The model under review builds one solid part; all positions refer to its coordinate system, in mm. Face numbers are marked on the shaded views. A direction names the side the tool comes from. Round coordinates to 2 decimals unless told otherwise and drop trailing zeros. Order: outer loops, then holes, each group sorted by start corner. A loop starts at its lowest first (then second) coordinate and runs counter-clockwise, first axis right, second up. Notation, with made-up numbers: (48, -6.5) - (70, -6.5) arc R28 ccw to (70, 24.5) - close; hole circle Ø10 at (37.5, 50). An arc over 180 degrees is marked (long way). One line per question, with ' | ' between items. Start each with the question number.
Item 1: Add section C-C on z = 8. State the section outline as (x, y) points.
Item 2: Insertion check: pin 1 Ø6.5 at (x, y) = (-1, 23.5) entering from +Z; pin 2 Ø2 at (y, z) = (4, 7) entering from -X; pin 3 Ø1.5 at (y, z) = (6, 5) entering from -X. Each pin has a flat end and moves straight along its axis. Give the tip position at first contact, or say it passes through.
Item 3: Add section A-A on x = 0. State the section outline as (y, z) points, and give its area (3 significant figures).
Item 4: Draft analysis for pull direction Z (two halves, no side actions). For the marked faces 1, 2 and 3, state which applies: +Z half, -Z half, draft (parallel to the pull), parting line (faces both ways), or undercut.
Item 5: For L1, parallel to Z at x = 5.7, y = 3.85; L2, parallel to Y at x = 3.5, z = 9; L3, parallel to Y at x = 4.25, z = 4, list the stretches that pass through material, from the lowest coordinate up. Write a range as [from, to].
Item 6: Add section D-D on y = 30. State the section outline as (x, z) points.
Item 7: Tool access review of the marked faces 4 and 5: name each direction out of +Z, -Z, +X, -X, +Y, -Y from which nothing blocks a thin tool from reaching the whole face with its end or side.
Autodesk Inventor part; units mm, degrees
ref_plane "YZ Plane" through (0, 0, 0) normal (1, 0, 0) x (0, 1, 0)
ref_plane "XZ Plane" through (0, 0, 0) normal (0, 1, 0) x (-1, 0, 0)
ref_plane "XY Plane" through (0, 0, 0) normal (0, 0, 1) x (1, 0, 0)
sketch "Sketch1" plane through (0, 0, 0) normal (0, 0, 1) x (1, 0, 0)
  circle A0 centre (0, 25) radius 4.1
  circle A1 centre (0, 25) radius 15
  line L0 (-14.9332, 23.5861) -> (-12.7, 0)
  line L1 (-12.7, 0) -> (0, 0)
  line L2 (0, 0) -> (0, 25)
  line L3 (14.9332, 23.5861) -> (12.7, 0)
  line L4 (12.7, 0) -> (0, 0)
  circle A2 centre (0, 25) radius 11.15
  point P0 (14.9332, 23.5861)
  dimension "d1" = 30
  dimension "d0" = 8.2
  dimension "d2" = 25.4
  dimension "d5" = 25
  dimension "d16" = 22.3
extrude "Extrusion1" add sketch "Sketch1" along normal blind 10 contours A2 | A1 | A1 L3 L4 L2 | L2 L1 L0 A1
sketch "Sketch2" plane through (-12.7, 0, 0) normal (0, -1, 0) x (1, 0, 0)
  line L0 (0, 0) -> (25.4, 0)
  line L1 (25.4, 0) -> (25.4, 10)
  line L2 (0, 10) -> (25.4, 10)
  line L3 (0, 0) -> (0, 10)
  circle A0 centre (7, 5) radius 1.65
  point P0 (12.7, 0)
  point P1 (0, 5)
  dimension "d6" = 3.3
  dimension "d7" = 7
extrude "Extrusion2" cut sketch "Sketch2" against normal blind 15 contours A0
ref_plane "Work Plane1" through (-12.7, 5, 0) normal (0, -1, 0) x (1, 0, 0)
sketch "Sketch3" plane through (-12.7, 5, 0) normal (0, -1, 0) x (1, 0, 0)
  circle A0 centre (7, 5) radius 1.65
  line L0 (9.9, 6.6743) -> (9.9, 3.3257)
  line L1 (9.9, 3.3257) -> (7, 1.6514)
  line L2 (7, 1.6514) -> (4.1, 3.3257)
  line L3 (4.1, 3.3257) -> (4.1, 6.6743)
  line L4 (4.1, 6.6743) -> (7, 8.3486)
  line L5 (7, 8.3486) -> (9.9, 6.6743)
  line L6 (4.1, 6.6743) -> (9.9, 6.6743)
  line L7 (9.9, 6.6743) -> (9.9, 13.9222)
  line L8 (9.9, 13.9222) -> (4.1, 13.9222)
  line L9 (4.1, 13.9222) -> (4.1, 6.6743)
  point P0 (12.7, 0)
  dimension "d11" = 5.8
extrude "Extrusion3" cut sketch "Sketch3" against normal blind 3
mirror "Mirror1" about plane through (0, 0, 0) normal (1, 0, 0) of "Extrusion3", "Extrusion2"
sketch "Sketch4" plane through (0, 0, 0) normal (0, 0, -1) x (-1, 0, 0)
  line L0 (12.7, 0) -> (-12.7, 0)
  line L1 (14.9332, 23.5861) -> (12.7, 0)
  arc A0 (14.9332, 23.5861) -> (-14.9332, 23.5861) centre (0, 25) ccw
  line L2 (-12.7, 0) -> (-14.9332, 23.5861)
  circle A1 centre (0, 25) radius 4.1
  point P0 (0, 0)
extrude "Extrusion4" add sketch "Sketch4" against normal blind 3 contours A1
sketch "Sketch5" plane through (0, 0, 10) normal (0, 0, 1) x (1, 0, 0)
  line L0 (8.6, 8) -> (8.6, 5)
  line L1 (8.6, 5) -> (2.8, 5)
  line L2 (2.8, 5) -> (2.8, 8)
  line L3 (2.8, 8) -> (8.6, 8)
  line L4 (-8.6, 5) -> (-8.6, 8)
  line L5 (-8.6, 8) -> (-2.8, 8)
  line L6 (-2.8, 8) -> (-2.8, 5)
  line L7 (-2.8, 5) -> (-8.6, 5)
  line L8 (-12.7, 0) -> (12.7, 0)
  line L9 (12.7, 0) -> (14.9332, 23.5861)
  arc A0 (14.9332, 23.5861) -> (-14.9332, 23.5861) centre (0, 25) ccw
  line L10 (-14.9332, 23.5861) -> (-12.7, 0)
  circle A1 centre (0, 25) radius 4.1
  circle A2 centre (0, 25) radius 4.1
  circle A3 centre (0, 25) radius 11.15
  point P0 (0, 0)
  dimension "d17" = 22.3
extrude "Extrusion5" cut sketch "Sketch5" against normal blind 7 contours A3
properties part number "OTRO_EXTREMO" material "Steel, Mild, Welded"
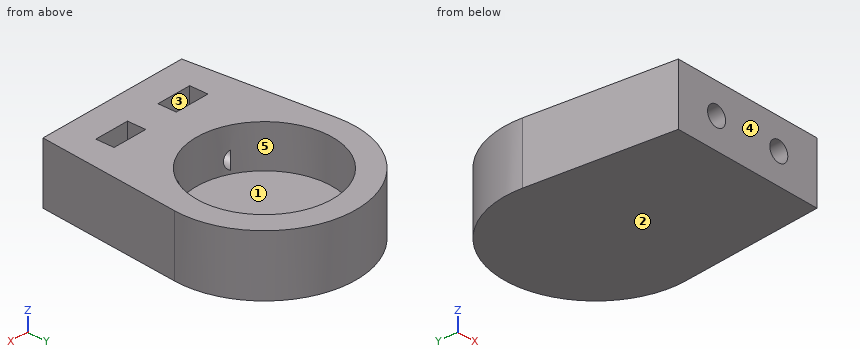
Determined:
1) outline: (-14.93, 23.59) - (-12.7, 0) - (12.7, 0) - (14.93, 23.59) arc R15 ccw (long way) to start; hole circle Ø22.3 at (0, 25); hole (-8.6, 5) - (-2.8, 5) - (-2.8, 8) - (-8.6, 8) - close; hole (2.8, 5) - (8.6, 5) - (8.6, 8) - (2.8, 8) - close
2) pin 1: z = 3 | pin 2: x = -13.17 | pin 3: x = -13.34
3) outline: (0, 0) - (40, 0) - (40, 10) - (36.15, 10) - (36.15, 3) - (13.85, 3) - (13.85, 10) - (0, 10) - close | area: 244 mm2
4) face 1: +Z half | face 2: -Z half | face 3: draft
5) L1: [0, 3.35], [6.65, 10] | L2: [0, 5], [8, 14.41], [35.59, 39.59] | L3: [0, 5], [8, 14.69], [35.31, 39.39]
6) outline: (-14.14, 0) - (14.14, 0) - (14.14, 10) - (9.97, 10) - (9.97, 3) - (-9.97, 3) - (-9.97, 10) - (-14.14, 10) - close
7) face 4: +Z, -Z, +X, -X, -Y | face 5: +Z
